Design review of the part built by this model. Coordinates are the model's own, in mm. Round coordinates to 2 decimals unless told otherwise and drop trailing zeros. Loops run counter-clockwise (first coordinate to the right, second up) from the corner with the lowest first, then second, coordinate; pieces in that order, holes last. Notation, with made-up numbers: (-39.75, -1) -> (-21.75, -1) arc R37 cw to (-21.75, 37) -> close; hole circle Ø5 at (69, -39.75). An arc over 180 degrees is marked (long way). Use a Markdown table: item, result. Add a question column.
from build123d import *

# Parameters (mm, degrees)
SKETCH2_R           = 1.65
SKETCH2_R_2         = 11
SKETCH2_R_3         = 2.25
BOSS_EXTRUDE1_DEPTH = 3.8


with BuildPart() as part:
    # Sketch2 → Boss-Extrude1 (new body)
    with BuildSketch(Plane.XY):
        with BuildLine():
            Line((-170.5, 150), (-137.4, 150))
            ThreePointArc((-137.4, 150), (-135.985786438, 149.414213562), (-135.4, 148))
            Line((-135.4, 148), (-135.4, 70))
            Line((-135.4, 70), (135.4, 70))
            Line((135.4, 70), (135.4, 148))
            ThreePointArc((135.4, 148), (135.985786438, 149.414213562), (137.4, 150))
            Line((137.4, 150), (170.5, 150))
            ThreePointArc((170.5, 150), (171.914213562, 149.414213562), (172.5, 148))
            Line((172.5, 148), (172.5, 67.8042249))
            Line((172.5, 67.8042249), (165.5, 67.8042249))
            Line((165.5, 67.8042249), (165.5, -17.8042249))
            Line((165.5, -17.8042249), (172.5, -17.8042249))
            Line((172.5, -17.8042249), (172.5, -99))
            ThreePointArc((172.5, -99), (172.207106781, -99.707106781), (171.5, -100))
            Line((171.5, -100), (137.4, -100))
            ThreePointArc((137.4, -100), (135.985786438, -99.414213562), (135.4, -98))
            Line((135.4, -98), (135.4, -22))
            ThreePointArc((135.4, -22), (134.814213562, -20.585786438), (133.4, -20))
            Line((133.4, -20), (-133.4, -20))
            ThreePointArc((-133.4, -20), (-134.814213562, -20.585786438), (-135.4, -22))
            Line((-135.4, -22), (-135.4, -98))
            ThreePointArc((-135.4, -98), (-135.985786438, -99.414213562), (-137.4, -100))
            Line((-137.4, -100), (-169.5, -100))
            ThreePointArc((-169.5, -100), (-171.621320344, -99.121320344), (-172.5, -97))
            Line((-172.5, -97), (-172.5, -17.8042249))
            Line((-172.5, -17.8042249), (-165.5, -17.8042249))
            Line((-165.5, -17.8042249), (-165.5, 67.8042249))
            Line((-165.5, 67.8042249), (-172.5, 67.8042249))
            Line((-172.5, 67.8042249), (-172.5, 148))
            ThreePointArc((-172.5, 148), (-171.914213562, 149.414213562), (-170.5, 150))
        make_face()
        with Locations(Location((-168.334802826, 116, 0), (0, 0, 180))):
            Circle(SKETCH2_R, mode=Mode.SUBTRACT)
        with Locations(Location((-139.665197174, 116, 0), (0, 0, 180))):
            Circle(SKETCH2_R, mode=Mode.SUBTRACT)
        with Locations(Location((168.334802826, 116, 0), (0, 0, 180))):
            Circle(SKETCH2_R, mode=Mode.SUBTRACT)
        with Locations(Location((139.665197174, 116, 0), (0, 0, 180))):
            Circle(SKETCH2_R, mode=Mode.SUBTRACT)
        with Locations(Location((154, 116, 0), (0, 0, 180))):
            Circle(SKETCH2_R_2, mode=Mode.SUBTRACT)
        with Locations(Location((-154, 116, 0), (0, 0, 180))):
            Circle(SKETCH2_R_2, mode=Mode.SUBTRACT)
        with Locations(Location((160.5, -0.5, 0), (0, 0, 180))):
            Circle(SKETCH2_R, mode=Mode.SUBTRACT)
        with Locations(Location((160.5, 50.5, 0), (0, 0, 180))):
            Circle(SKETCH2_R, mode=Mode.SUBTRACT)
        with Locations(Location((-160.5, -0.5, 0), (0, 0, 180))):
            Circle(SKETCH2_R, mode=Mode.SUBTRACT)
        with Locations(Location((-160.5, 50.5, 0), (0, 0, 180))):
            Circle(SKETCH2_R, mode=Mode.SUBTRACT)
        with Locations(Location((-35, 10.055, 0), (0, 0, 180))):
            Circle(SKETCH2_R_3, mode=Mode.SUBTRACT)
        with Locations(Location((-35, 39.945, 0), (0, 0, 180))):
            Circle(SKETCH2_R_3, mode=Mode.SUBTRACT)
        with Locations(Location((-59.06, 39.945, 0), (0, 0, 180))):
            Circle(SKETCH2_R_3, mode=Mode.SUBTRACT)
        with Locations(Location((-59.06, 10.055, 0), (0, 0, 180))):
            Circle(SKETCH2_R_3, mode=Mode.SUBTRACT)
        with Locations(Location((59.06, 10.055, 0), (0, 0, 180))):
            Circle(SKETCH2_R_3, mode=Mode.SUBTRACT)
        with Locations(Location((35, 10.055, 0), (0, 0, 180))):
            Circle(SKETCH2_R_3, mode=Mode.SUBTRACT)
        with Locations(Location((35, 39.945, 0), (0, 0, 180))):
            Circle(SKETCH2_R_3, mode=Mode.SUBTRACT)
        with Locations(Location((59.06, 39.945, 0), (0, 0, 180))):
            Circle(SKETCH2_R_3, mode=Mode.SUBTRACT)
        with Locations(Location((168.334802826, -66, 0), (0, 0, 180))):
            Circle(SKETCH2_R, mode=Mode.SUBTRACT)
        with Locations(Location((139.665197174, -66, 0), (0, 0, 180))):
            Circle(SKETCH2_R, mode=Mode.SUBTRACT)
        with Locations(Location((154, -66, 0), (0, 0, 180))):
            Circle(SKETCH2_R_2, mode=Mode.SUBTRACT)
        with Locations(Location((-154, -66, 0), (0, 0, 180))):
            Circle(SKETCH2_R_2, mode=Mode.SUBTRACT)
        with Locations(Location((-139.665197174, -66, 0), (0, 0, 180))):
            Circle(SKETCH2_R, mode=Mode.SUBTRACT)
        with Locations(Location((-168.334802826, -66, 0), (0, 0, 180))):
            Circle(SKETCH2_R, mode=Mode.SUBTRACT)
        with BuildLine():
            Line((-72.45742566, 62.171403079), (-118.05517368, 62.171403079))
            ThreePointArc((-118.05517368, 62.171403079), (-120.883600805, 60.999830204), (-122.05517368, 58.171403079))
            Line((-122.05517368, 58.171403079), (-122.05517368, -8.171403079))
            ThreePointArc((-122.05517368, -8.171403079), (-120.883600805, -10.999830204), (-118.05517368, -12.171403079))
            Line((-118.05517368, -12.171403079), (-72.45742566, -12.171403079))
            ThreePointArc((-72.45742566, -12.171403079), (-69.628998535, -10.999830204), (-68.45742566, -8.171403079))
            Line((-68.45742566, -8.171403079), (-68.45742566, 58.171403079))
            ThreePointArc((-68.45742566, 58.171403079), (-69.628998535, 60.999830204), (-72.45742566, 62.171403079))
        make_face(mode=Mode.SUBTRACT)
        with BuildLine():
            Line((72.45742566, 62.171403079), (118.05517368, 62.171403079))
            ThreePointArc((118.05517368, 62.171403079), (120.883600805, 60.999830204), (122.05517368, 58.171403079))
            Line((122.05517368, 58.171403079), (122.05517368, -8.171403079))
            ThreePointArc((122.05517368, -8.171403079), (120.883600805, -10.999830204), (118.05517368, -12.171403079))
            Line((118.05517368, -12.171403079), (72.45742566, -12.171403079))
            ThreePointArc((72.45742566, -12.171403079), (69.628998535, -10.999830204), (68.45742566, -8.171403079))
            Line((68.45742566, -8.171403079), (68.45742566, 58.171403079))
            ThreePointArc((68.45742566, 58.171403079), (69.628998535, 60.999830204), (72.45742566, 62.171403079))
        make_face(mode=Mode.SUBTRACT)
    extrude(amount=BOSS_EXTRUDE1_DEPTH)


solid = part.part
1. Mouldability with a two-part tool opening along Y and no side actions: class faces 1 (the face through (165, 116, 2)), 2 (the face through (1, 16, 3.8)) as +Y half, -Y half, draft (parallel to the pull), parting line (faces both ways), or undercut.
2. Consider section B-B on y = -38.5. State the section outline as (x, z) points.
3. To check wall thickness, follow probe 1 along X at (y, z) = (34, 3.65); probe 2 along Y at (x, z) = (-59.06, 2) (3 decimals); probe 3 along X at (y, z) = (-2, 0.6). State the ranges of each line that lie inside material, in increasing order. Write a range as from..to.
4. Consider section D-D on z = 2.35. Give the number of separate pieces and of enclosed holes in the cut face, plus the area to 3 significant figures.
5. Consider section C-C on x = -51.5. State the section outline as (y, z) points.
6. Consider section A-A on y = 29. State the section outline as (x, z) points, plus the area to 3 significant figures.
7. Insertion check: P1, Ø2, axis at x = -51.5, z = 2, coming from the -Y side; P2, Ø1.9, axis at x = 105.5, z = 2, coming from the +Y side; P3, Ø1.1, axis at y = 13.5, z = 2.5, coming from the -X side. Each pin has a flat end and moves straight along its axis. Give the tip position at first contact, or say it passes through.
Verdict:
| question | item | result |
|---|---|---|
| 1 | face 1 | undercut |
| 1 | face 2 | draft |
| 2 | outline | (-172.5, 0) -> (-135.4, 0) -> (-135.4, 3.8) -> (-172.5, 3.8) -> close; (135.4, 0) -> (172.5, 0) -> (172.5, 3.8) -> (135.4, 3.8) -> close |
| 3 | probe 1 | x = -165.5..-122.06, -68.46..68.46, 122.06..165.5 |
| 3 | probe 2 | y = -20..7.805, 12.305..37.695, 42.195..70 |
| 3 | probe 3 | x = -165.5..-161.19, -159.81..-122.06, -68.46..68.46, 122.06..159.81, 161.19..165.5 |
| 4 | separate pieces | 1 |
| 4 | enclosed holes | 26 |
| 4 | area | 32,000 mm² |
| 5 | outline | (-20, 0) -> (70, 0) -> (70, 3.8) -> (-20, 3.8) -> close |
| 6 | outline | (-165.5, 0) -> (-122.06, 0) -> (-122.06, 3.8) -> (-165.5, 3.8) -> close; (-68.46, 0) -> (68.46, 0) -> (68.46, 3.8) -> (-68.46, 3.8) -> close; (122.06, 0) -> (165.5, 0) -> (165.5, 3.8) -> (122.06, 3.8) -> close |
| 6 | area | 850 mm² |
| 7 | P1 | stops at y = -20 |
| 7 | P2 | stops at y = 70 |
| 7 | P3 | stops at x = -165.5 |
